Design review of the part shown in the three views and the two pictorial views. Dimensions are in mm from the part's minimum x, y and z. A direction names the side the tool comes from. Coordinates: 2 decimals unless noted, no trailing zeros. Write each loop counter-clockwise with the first axis right and the second up, starting at its lowest first coordinate (ties: lowest second). Pieces come first, ordered by that corner, then holes.
Q1. For pin 1 Ø4 at (x, y) = (2, 20.5) entering from -Z; pin 2 Ø6 at (y, z) = (22.5, 1.5) entering from +X; pin 3 Ø3 at (x, y) = (10, 19) entering from +Z, all flat-tipped, find the tip position at first contact; note any pin that passes through.
Q2. Take a section at A-A, the plane z = 6.25. Write out the cut boundary in (x, y).
Q3. For L1, parallel to Y at x = 10.75, z = 2.5; L2, parallel to X at y = 22.5, z = 4.25; L3, parallel to X at y = 19.5, z = 7, list the stretches that pass through material, from the lowest coordinate up.
Q4. The part is to be moulded in two halves that separate along Y. For the marked faces 1, 2 and 3, say which applies: released by +Y, released by -Y, zero draft, split by the parting line, or undercut.
Q5. Take a section at C-C, the plane y = 10. Write out the cut boundary in (x, z).
Q6. For the marked faces 4, 5 and 6, list the 3-axis set-ups (+Z, -Z, +X, -X, +Y, -Y) from which the entire face can be reached by the end or side of a thin tool; tool diameter is ignored.
Q7. Take a section at D-D, the plane z = 8.75. Write out the cut boundary in (x, y), plus the area to 3 significant figures.
Q8. Take a section at B-B, the plane x = 6.7. Write out the cut boundary in (y, z), plus the area to 3 significant figures.
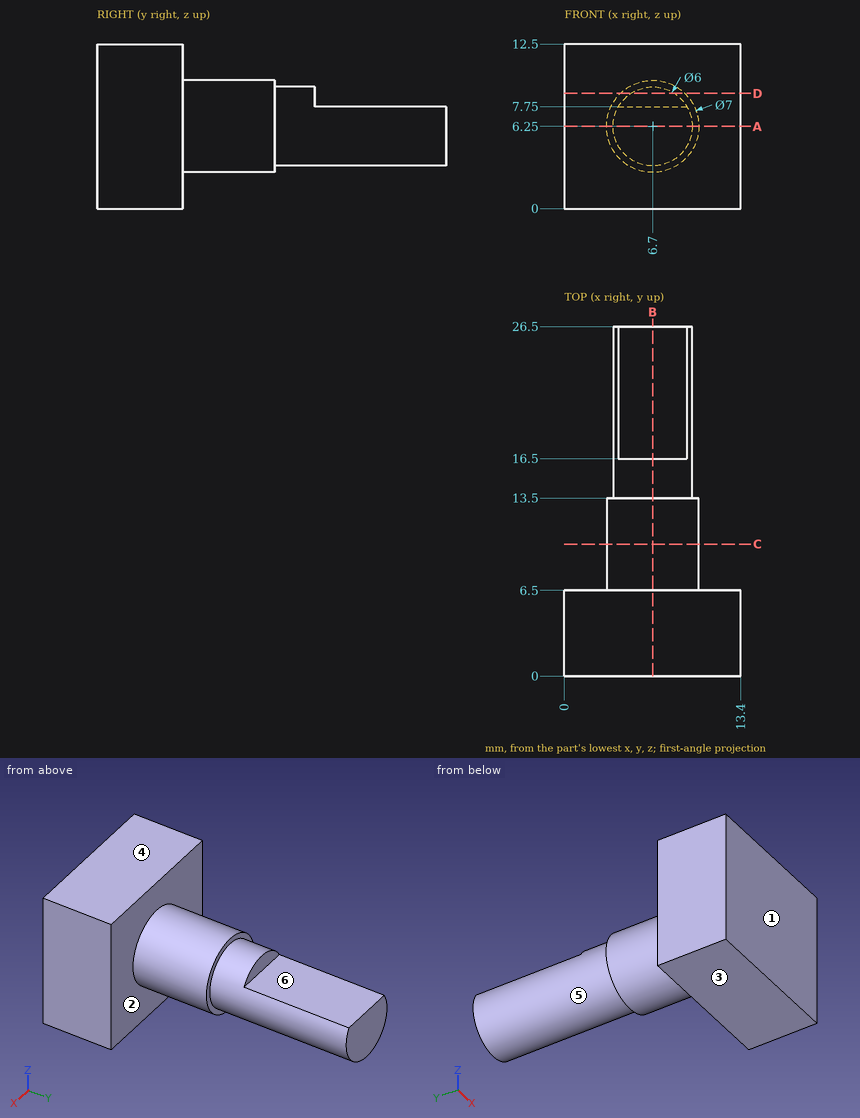
Responses:
1. pin 1: stops at z = 4.94
1. pin 2: stops at x = 9.14
1. pin 3: stops at z = 7.75
2. outline: (0, 0) - (13.4, 0) - (13.4, 6.5) - (10.2, 6.5) - (10.2, 13.5) - (9.7, 13.5) - (9.7, 26.5) - (3.7, 26.5) - (3.7, 13.5) - (3.2, 13.5) - (3.2, 6.5) - (0, 6.5) - close
3. L1: y = 0 to 6.5
3. L2: x = 4.46 to 8.94
3. L3: x = 3.8 to 9.6
4. face 1: released by -Y
4. face 2: released by +Y
4. face 3: zero draft
5. outline: circle Ø7 at (6.7, 6.25)
6. face 4: +Z, +X, -X, +Y, -Y
6. face 5: +Y
6. face 6: +Z, +X, -X, +Y
7. outline: (0, 0) - (13.4, 0) - (13.4, 6.5) - (9.15, 6.5) - (9.15, 13.5) - (8.36, 13.5) - (8.36, 16.5) - (5.04, 16.5) - (5.04, 13.5) - (4.25, 13.5) - (4.25, 6.5) - (0, 6.5) - close
7. area: 131 mm2
8. outline: (0, 0) - (6.5, 0) - (6.5, 2.75) - (13.5, 2.75) - (13.5, 3.25) - (26.5, 3.25) - (26.5, 7.75) - (16.5, 7.75) - (16.5, 9.25) - (13.5, 9.25) - (13.5, 9.75) - (6.5, 9.75) - (6.5, 12.5) - (0, 12.5) - close
8. area: 193 mm2
